from build123d import *

# Parameters (mm, degrees)
F0_W      = 163.322
F0_H      = 72.898
F1_DEPTH  = 7.366
F2_R      = 7.62
F3_R      = 5.08
F4_T      = -2.54
F5_R      = 10.5491920508
F6_DEPTH  = 30.48
F4_FACE_R = 10.5491920508
F7_DEPTH  = 25.4


with BuildPart() as f1:
    # F0 (on Top) → F1 (new body)
    with BuildSketch(Plane.XY):
        with Locations((81.661, 36.449)):
            Rectangle(F0_W, F0_H)
    extrude(amount=F1_DEPTH)

    # F2
    f2_edges = [f1.edges().sort_by_distance(p)[0] for p in [
        (163.322, 72.898, 3.683),
        (0, 72.898, 3.683),
        (163.322, 0, 3.683),
        (0, 0, 3.683),
    ]]
    fillet(f2_edges, radius=F2_R)

    # F3
    f3_edges = [f1.edges().sort_by_distance(p)[0] for p in [
        (0, 36.449, 0),
        (2.231846, 70.666154, 0),
        (2.231846, 2.231846, 0),
        (81.661, 72.898, 0),
        (81.661, 0, 0),
        (161.090154, 70.666154, 0),
        (161.090154, 2.231846, 0),
        (163.322, 36.449, 0),
    ]]
    fillet(f3_edges, radius=F3_R)

    # F4
    f4_openings = [f1.faces().sort_by_distance(p)[0] for p in [
        (81.661, 36.449, 7.366),
    ]]
    offset(amount=F4_T, openings=f4_openings)

    # F5 (on Top) → F6 (cut)
    with BuildSketch(Plane.XY):
        with Locations((37.9090681672, 25.489339605)):
            Circle(F5_R)
    extrude(amount=F6_DEPTH, mode=Mode.SUBTRACT)

    # F5 (on Top) + F4_face (on face) → F7 (join)
    with BuildSketch(Plane.XY):
        with Locations((37.9090681672, 25.489339605)):
            Circle(F5_R)
    with BuildSketch(Plane(origin=(83.3139491245, 36.8630562553, 2.54), x_dir=(1, 0, 0), z_dir=(0, 0, 1))):
        with BuildLine():
            Line((-78.2339491245, 28.4149437447), (-78.2339491245, -29.2430562553))
            ThreePointArc((-78.2339491245, -29.2430562553), (-77.4900003487, -31.0391074795), (-75.6939491245, -31.7830562553))
            Line((-75.6939491245, -31.7830562553), (72.3880508755, -31.7830562553))
            ThreePointArc((72.3880508755, -31.7830562553), (74.1841020997, -31.0391074795), (74.9280508755, -29.2430562553))
            Line((74.9280508755, -29.2430562553), (74.9280508755, 28.4149437447))
            ThreePointArc((74.9280508755, 28.4149437447), (74.1841020997, 30.210994969), (72.3880508755, 30.9549437447))
            Line((72.3880508755, 30.9549437447), (-75.6939491245, 30.9549437447))
            ThreePointArc((-75.6939491245, 30.9549437447), (-77.4900003487, 30.210994969), (-78.2339491245, 28.4149437447))
        make_face()
        with Locations((-45.4048809573, -11.3737166503)):
            Circle(F4_FACE_R, mode=Mode.SUBTRACT)
    extrude(amount=-F7_DEPTH)


solid = f1.part
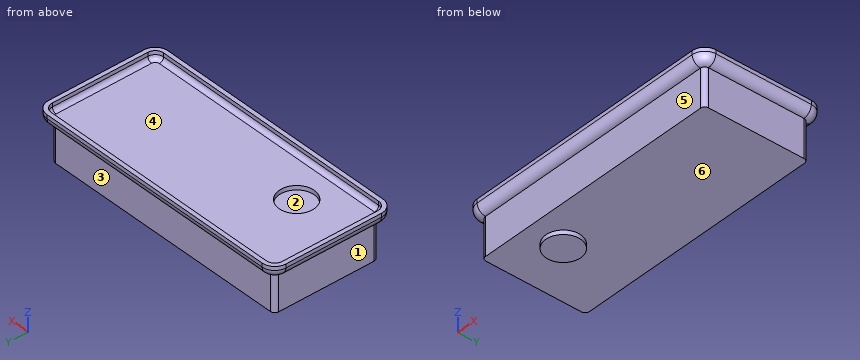
Part model, mm, in its own coordinate system. Face numbers are marked on the shaded views. A direction names the side the tool comes from. Round coordinates to 2 decimals unless told otherwise and drop trailing zeros. Order: outer loops, then holes, each group sorted by start corner. A loop starts at its lowest first (then second) coordinate and runs counter-clockwise, first axis right, second up. Notation, with made-up numbers: (65, 3) -> (119, 3) arc R17 cw to (119, 20) -> close; hole circle Ø2 at (-37, -26.5). An arc over 180 degrees is marked (long way). Put each result on its own line as item: value.
Q1. Pin check, flat tips, straight feed: pin 1 Ø5 at (x, y) = (35.5, 25) entering from +Z; pin 2 Ø1.5 at (x, y) = (38, 11) entering from -Z; pin 3 Ø12 at (x, z) = (83.5, -7) entering from -Y. Stop position of each tip, or through.
From the geometry:
pin 1: stops at z = 0
pin 2: stops at z = -22.86
pin 3: stops at y = 5.08
Q2. Wall check: line 1 (X direction, y = 48, z = 5); line 2 (Y direction, x = 46, z = -22.5); line 3 (X direction, y = 46, z = -20). Give the ranges that are in metal, low to high. Write a range as [from, to].
From the geometry:
line 1: x = [0, 2.54], [160.78, 163.32]
line 2: y = [5.08, 67.82]
line 3: x = [5.08, 158.24]
Q3. Band-saw the part on A-A (z = -21). Give the cut face in (x, y), and give its area (3 significant figures).
From the geometry:
outline: (5.08, 7.62) arc R2.54 ccw to (7.62, 5.08) -> (155.7, 5.08) arc R2.54 ccw to (158.24, 7.62) -> (158.24, 65.28) arc R2.54 ccw to (155.7, 67.82) -> (7.62, 67.82) arc R2.54 ccw to (5.08, 65.28) -> close
area: 9,600 mm2
Q4. Band-saw the part on B-B (x = 25). Give the cut face in (y, z), and give its area (3 significant figures).
From the geometry:
outline: (0, 5.08) arc R5.08 ccw to (5.08, 0) -> (5.08, -22.86) -> (67.82, -22.86) -> (67.82, 0) arc R5.08 ccw to (72.9, 5.08) -> (72.9, 7.37) -> (70.36, 7.37) -> (70.36, 5.08) arc R2.54 cw to (67.82, 2.54) -> (5.08, 2.54) arc R2.54 cw to (2.54, 5.08) -> (2.54, 7.37) -> (0, 7.37) -> close
area: 1,640 mm2
Q5. Band-saw the part on C-C (y = 16.5). Give the cut face in (x, z).
From the geometry:
outline: (0, 5.08) arc R5.08 ccw to (5.08, 0) -> (5.08, -22.86) -> (32.39, -22.86) -> (32.39, -25.4) -> (43.43, -25.4) -> (43.43, -22.86) -> (158.24, -22.86) -> (158.24, 0) arc R5.08 ccw to (163.32, 5.08) -> (163.32, 7.37) -> (160.78, 7.37) -> (160.78, 5.08) arc R2.54 cw to (158.24, 2.54) -> (43.43, 2.54) -> (43.43, 0) -> (32.39, 0) -> (32.39, 2.54) -> (5.08, 2.54) arc R2.54 cw to (2.54, 5.08) -> (2.54, 7.37) -> (0, 7.37) -> close
Q6. Tool access for the marked faces 1, 2 and 3: list every direction of +Z, -Z, +X, -X, +Y, -Y with a clear straight run to the whole face (end or side of a thin tool).
From the geometry:
face 1: -Z, -X, +Y, -Y
face 2: +Z
face 3: -Z, +X, -X, +Y
Q7. Pull direction Y, two halves, no side cores. Call the marked faces 4, 5 and 6: pulls with the +Y half, pulls with the -Y half, needs draft (parallel to the pull), parting line crosses it, or undercut.
From the geometry:
face 4: undercut
face 5: pulls with the -Y half
face 6: needs draft
